Verification items for the finished model (mm, model axes). Face numbers are marked on the shaded views. A direction names the side the tool comes from. Coordinates: 2 decimals unless noted, no trailing zeros. Write each loop counter-clockwise with the first axis right and the second up, starting at its lowest first coordinate (ties: lowest second). Pieces come first, ordered by that corner, then holes. Notation, with made-up numbers: (75.25, 79) -> (116.25, 79) arc R18 cw to (116.25, 104) -> close; hole circle Ø3 at (34, -35.5). An arc over 180 degrees is marked (long way). Use CSV: the item, a comma, the result in double quotes.
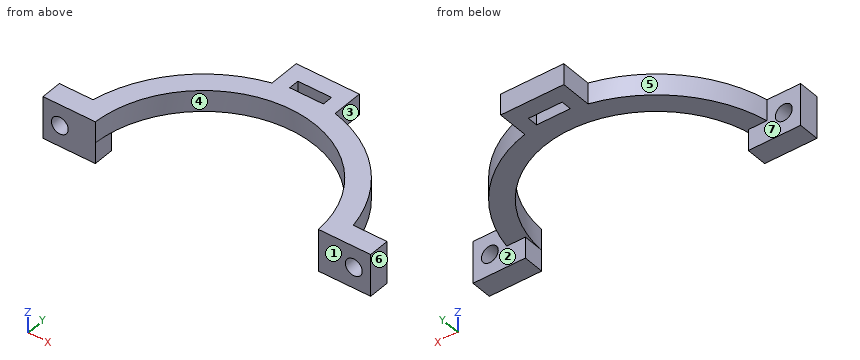
Autodesk Inventor part; units mm, degrees
ref_plane "YZ Plane" through (0, 0, 0) normal (1, 0, 0) x (0, 1, 0)
ref_plane "Work Plane1" through (0, 0, -3.5) normal (0, 0, 1) x (1, 0, 0)
sketch "Sketch1" plane through (0, 0, -3.5) normal (0, 0, 1) x (1, 0, 0)
  circle A0 centre (0, 0) radius 26.5
  circle A1 centre (0, 0) radius 31.5
  point P0 (0, 0)
  dimension "d1" = 5
extrude "Extrusion1" add sketch "Sketch1" against normal blind 5
sketch "Sketch5" plane through (0, 0, 0) normal (1, 0, 0) x (0, 1, 0)
  line L0 (6.0883, 0) -> (4.0883, 0)
  line L1 (4.0883, 0) -> (4.0883, -15.2563)
  line L2 (4.0883, -15.2563) -> (6.0883, -15.2563)
  line L3 (6.0883, -15.2563) -> (6.0883, 0)
  line L4 (-1, 2.6587) -> (1, 2.6587)
  line L5 (1, 2.6587) -> (1, -12.1151)
  line L6 (1, -12.1151) -> (-1, -12.1151)
  line L7 (-1, -12.1151) -> (-1, 2.6587)
  point P0 (0, 0)
  dimension "d4" = 2
  dimension "d5" = 2
  dimension "d6" = 1
extrude "Extrusion2" cut sketch "Sketch5" along normal through all both and the other way through all contours L4 L5 L6 L7
sketch "Sketch6" plane through (0, 0, -8.5) normal (0, 0, -1) x (-1, 0, 0)
  line L0 (26.4811, 1) -> (31.4841, 1)
  line L1 (-31.4841, 1) -> (-26.4811, 1)
  arc A0 (26.4811, 1) -> (-26.4811, 1) centre (0, 0) ccw
  line L2 (26.4811, 1) -> (31.4841, 1)
  arc A1 (31.4841, 1) -> (-31.4841, 1) centre (0, 0) ccw
  line L3 (-53.7275, 6) -> (74.5535, 6)
  line L4 (26.4811, 1) -> (30.9233, 1)
  line L5 (30.9233, 1) -> (30.9233, 6)
  line L6 (30.9233, 6) -> (26.4811, 6)
  line L7 (26.4811, 6) -> (26.4811, 1)
  dimension "d9" = 5
extrude "Extrusion3" add sketch "Sketch6" along normal blind 5 contours L7 L3 L5 L0
sketch "Sketch7" plane through (-30.9233, 1, -8.5) normal (-1, 0, 0) x (0, 0, 1)
  line L0 (0, 5) -> (0, 0)
  line L1 (0, 5) -> (-5, 5)
  line L2 (-5, 0) -> (-5, 5)
  line L3 (0, 0) -> (-5, 0)
  point P0 (8.5, -1)
extrude "Extrusion4" add sketch "Sketch7" along normal blind 5
sketch "Sketch8" plane through (-35.9233, 6, -8.5) normal (0, 0, 1) x (1, 0, 0)
  arc A0 (5, 0) -> (4.4392, -5) centre (35.9233, -6) ccw
  line L0 (5, 0) -> (0, 0)
  line L1 (0, -5) -> (0, 0)
  line L2 (4.4392, -5) -> (0, -5)
extrude "Extrusion5" add sketch "Sketch8" along normal blind 5
sketch "Sketch9" plane through (-35.9233, 1, -8.5) normal (-1, 0, 0) x (0, 0, 1)
  line L0 (-5, 5) -> (5, 5)
  line L1 (-5, 5) -> (-5, 0)
  line L2 (-5, 0) -> (5, 0)
  line L3 (5, 5) -> (5, 0)
  point P0 (8.5, -1)
extrude "Extrusion6" add sketch "Sketch9" along normal blind 3
sketch "Sketch10" plane through (-30.9233, 6, -8.5) normal (0, 1, 0) x (1, 0, 0)
  circle A0 centre (-4, 0) radius 2
  point P0 (30.9233, -8.5)
  dimension "d18" = 4
extrude "Extrusion7" cut sketch "Sketch10" against normal up to next
mirror "Mirror1" about plane through (0, 0, 0) normal (1, 0, 0) of "Extrusion3", "Extrusion4", "Extrusion5", "Extrusion6", "Extrusion7"
sketch "Sketch11" plane through (0, 0, -8.5) normal (0, 0, -1) x (-1, 0, 0)
  line L0 (31.4841, -1) -> (26.4811, -1)
  arc A0 (-26.4811, -1) -> (26.4811, -1) centre (0, 0) ccw
  line L1 (-26.4811, -1) -> (-31.4841, -1)
  arc A1 (-31.4841, -1) -> (31.4841, -1) centre (0, 0) ccw
extrude "Extrusion8" cut sketch "Sketch11" against normal through all
ref_plane "Work Plane2" through (0, 35, 0) normal (0, 1, 0) x (-1, 0, 0)
sketch "Sketch12" plane through (0, 35, 0) normal (0, 1, 0) x (-1, 0, 0)
  line L0 (-30.9233, -3.5) -> (30.9233, -3.5) construction
  line L1 (-30.9233, -8.5) -> (30.9233, -8.5) construction
  line L2 (-7.5, -3.5) -> (7.5, -3.5)
  line L3 (7.5, -3.5) -> (7.5, -8.5)
  line L4 (7.5, -8.5) -> (-7.5, -8.5)
  line L5 (-7.5, -8.5) -> (-7.5, -3.5)
  point P0 (0, 0)
  dimension "d24" = 15
  dimension "d25" = 7.5
extrude "Extrusion9" add sketch "Sketch12" against normal up to next
sketch "Sketch13" plane through (0, 35, 0) normal (0, 1, 0) x (1, 0, 0)
  line L0 (7.5, 3.5) -> (-7.5, 3.5)
  line L1 (7.5, 8.5) -> (7.5, 3.5)
  line L2 (-7.5, 8.5) -> (7.5, 8.5)
  line L3 (-7.5, 3.5) -> (-7.5, 8.5)
  point P0 (0, 0)
extrude "Extrusion10" add sketch "Sketch13" along normal blind 3
sketch "Sketch14" plane through (0, 0, -8.5) normal (0, 0, -1) x (-1, 0, 0)
  line L0 (-7.5, 38) -> (7.5, 38)
  arc A0 (-7.5, 30.5941) -> (-30.9233, 6) centre (0, 0) ccw
  line L1 (-4, 34) -> (4, 34)
  line L2 (4, 34) -> (4, 31.5)
  line L3 (4, 31.5) -> (-4, 31.5)
  line L4 (-4, 31.5) -> (-4, 34)
  dimension "d30" = 8
  dimension "d31" = 2.5
  dimension "d32" = 4
  dimension "d33" = 4
extrude "Extrusion11" cut sketch "Sketch14" against normal blind 5
properties part number "CanBracket"
1) Scan lines: L1, parallel to X at y = 4, z = -12.5; L2, parallel to Z at x = -9.5, y = 26; L3, parallel to Y at x = -30.5, z = -12.75. Record each from-to range of solid material in increasing order.
Return value:
L1,"-38.92 to -26.48, 26.48 to 38.92"
L2,"-8.5 to -3.5"
L3,"1 to 6"
2) Set-up check for the marked faces 1, 2 and 3: record each of +Z, -Z, +X, -X, +Y, -Y from which the full face is reachable in a straight line by a thin tool's end or side.
Return value:
face 1,"+Z, -Z, +X, -X, -Y"
face 2,"-Z, +X, +Y"
face 3,"+Z, -Z, +X, +Y"
3) Gauge pin test, flat ends, axial feed: pin 1 (4 mm diameter, centred on x = -2.5, z = -8.5, fed in from -Y); pin 2 (11 mm diameter, centred on x = -15, y = 28, fed in from -Z); pin 3 (2 mm diameter, centred on y = 33.5, z = -5, fed in from -X). Record the tip position at first contact, or that the pin passes through.
Return value:
pin 1,"y = 26.12"
pin 2,"z = -8.5"
pin 3,"x = -7.5"
4) Cross-section at A-A (x = 0). Record the boundary of the cut face in (y, z), plus the area to 3 significant figures.
Return value:
outline,"(26.5, -8.5) -> (31.5, -8.5) -> (31.5, -3.5) -> (26.5, -3.5) -> close; (34, -8.5) -> (38, -8.5) -> (38, -3.5) -> (34, -3.5) -> close"
area,"45.0 mm2"
5) Cross-section at D-D (x = -18). Record the boundary of the cut face in (y, z), plus the area to 3 significant figures.
Return value:
outline,"(19.45, -8.5) -> (25.85, -8.5) -> (25.85, -3.5) -> (19.45, -3.5) -> close"
area,"32.0 mm2"
6) Mould release check, pull along X, two halves, no side actions. Record for the marked faces 4, 5, 6 and 7: released by +X, released by -X, zero draft, split by the parting line, or undercut.
Return value:
face 4,"undercut"
face 5,"released by -X"
face 6,"released by +X"
face 7,"zero draft"
7) Cross-section at B-B (y = 24.5). Record the boundary of the cut face in (x, z).
Return value:
outline,"(-19.8, -8.5) -> (-10.1, -8.5) -> (-10.1, -3.5) -> (-19.8, -3.5) -> close; (10.1, -8.5) -> (19.8, -8.5) -> (19.8, -3.5) -> (10.1, -3.5) -> close"
8) Cross-section at C-C (x = 24). Record the boundary of the cut face in (y, z), plus the area to 3 significant figures.
Return value:
outline,"(11.24, -8.5) -> (20.4, -8.5) -> (20.4, -3.5) -> (11.24, -3.5) -> close"
area,"45.8 mm2"
